Geometry: final body of the model. Coordinates: model frame, mm. Face numbers are marked on the shaded views. A direction names the side the tool comes from. Give positions to 0.01 mm unless a question says otherwise; leave off trailing zeros. Loops run counter-clockwise (first coordinate to the right, second up) from the corner with the lowest first, then second, coordinate; pieces in that order, holes last. Notation, with made-up numbers: (20.5, 40.25) - (69.5, 40.25) arc R16 ccw to (69.5, 63.25) - close; hole circle Ø9 at (55, 82.25). An arc over 180 degrees is marked (long way). Answer in a Markdown table with one row per item.
Solid Edge part; units mm, degrees
sketch "Sketch1" plane through (0, 0, 0) normal (0, -1, 0) x (1, 0, 0)
  circle A0 centre (0, 0) radius 21
extrude "Protrusion1" add sketch "Sketch1" along normal blind 20
sketch "Sketch2" plane through (0, 0, 0) normal (0, -1, 0) x (1, 0, 0)
  circle A0 centre (0, 0) radius 8
extrude "ExtrudedCutout_1" cut sketch "Sketch2" along normal blind 161.3
sketch "Sketch3" plane through (0, 0, 0) normal (0, -1, 0) x (1, 0, 0)
  circle A0 centre (0, 0) radius 16
  circle A1 centre (0, 0) radius 8
extrude "ExtrudedCutout_2" cut sketch "Sketch3" along normal blind 10
sketch "Sketch4" plane through (0, -10, -21) normal (0, 0, -1) x (0, 1, 0)
  circle A0 centre (5, 0) radius 2.5
extrude "Cutout1" cut sketch "Sketch4" against normal up to vertex (21 mm away)
pattern_circular "Pattern1" count 2 over 84.153 about axis through (-0.000024, 0, 0) along (0, 1, 0) of "Cutout1"
sketch "Sketch5" plane through (0, -20, 0) normal (0, -1, 0) x (0, 0, 1)
  circle A0 centre (0, 0) radius 8.35
extrude "Cutout2" cut sketch "Sketch5" against normal blind 63.3
sketch "Sketch6" plane through (-14.849242, -10, -14.849242) normal (-0.7071068, 0, -0.7071068) x (0, 1, 0)
  circle A0 centre (-5, 0) radius 2.25
extrude "ExtrudedCutout_9" cut sketch "Sketch6" against normal blind 20.6
sketch "Sketch7" plane through (-14.849242, -10, -14.849242) normal (-0.7071068, 0, -0.7071068) x (0, 1, 0)
  circle A0 centre (-5, 0) radius 2.25
  circle A1 centre (-5, 0) radius 4.5
extrude "ExtrudedCutout_10" cut sketch "Sketch7" against normal blind 4
chamfer "Chamfer_4" distance 6.98968 angle 45 1 edges at (-21, -20, 0)
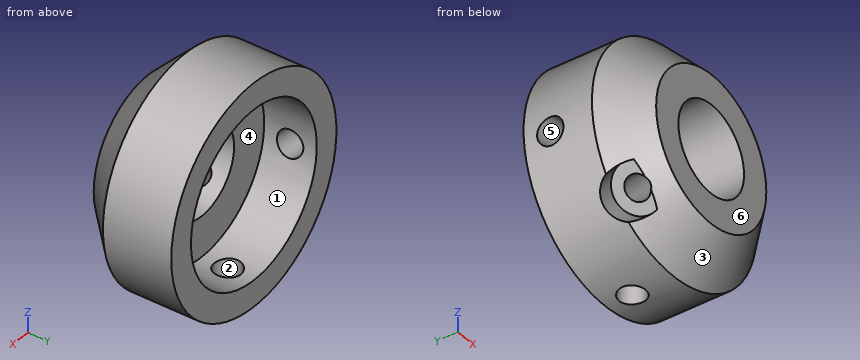
Q1. Cut plane A-A (x = 0). Output: boundary loops of the cut face in (y, z), and give its area (3 significant figures).
Check values:
| item | result |
|---|---|
| outline | (-20, -14.01) - (-13.01, -21) - (-7.5, -21) - (-7.5, -16) - (-10, -16) - (-10, -8.35) - (-20, -8.35) - close; (-20, 8.35) - (-10, 8.35) - (-10, 16) - (0, 16) - (0, 21) - (-13.01, 21) - (-20, 14.01) - close; (-2.5, -21) - (0, -21) - (0, -16) - (-2.5, -16) - close |
| area | 279 mm² |
Q2. Cut plane B-B (y = -5). Output: boundary loops of the cut face in (x, z), and give its area (3 significant figures).
Check values:
| item | result |
|---|---|
| outline | (-21, 0.36) - (-15.98, 0.88) arc R16 cw (long way) to (2.5, -15.8) - (2.5, -20.85) arc R21 ccw (long way) to start; (-20.49, -4.61) arc R21 ccw to (-2.5, -20.85) - (-2.5, -15.8) arc R16 cw to (-15.47, -4.1) - close |
| area | 531 mm² |
Q3. Cut plane D-D (z = 0). Give the number of separate pieces and of enclosed holes in the cut face, and give its area (3 significant figures).
Check values:
| item | result |
|---|---|
| separate pieces | 3 |
| enclosed holes | 0 |
| area | 288 mm² |
Q4. First-contact query: pin 1 (1.5 mm diameter, centred on x = 10.5, y = -12.5, fed in from +Z); pin 2 (16 mm diameter, centred on x = 7.5, z = -1, fed in from +Y); pin 3 (5 mm diameter, centred on y = -4.5, z = 5.5, fed in from -X). Flat tips, straight axial feed; report the tip coordinate or a pass-through.
Check values:
| item | result |
|---|---|
| pin 1 | z = 18.6 |
| pin 2 | y = -10 |
| pin 3 | x = -20.78 |
Q5. Reachability of the marked faces 1, 2 and 3 from +Z, -Z, +X, -X, +Y, -Y: full face, straight path, thin tool, end or side. Return the list, or none.
Check values:
| item | result |
|---|---|
| face 1 | +Y |
| face 2 | -Z |
| face 3 | -Y |
Q6. Draft query along Y for the marked faces 4, 5 and 6. Return one class per face: pulls with the +Y half, pulls with the -Y half, needs draft (parallel to the pull), parting line crosses it, or undercut.
Check values:
| item | result |
|---|---|
| face 4 | pulls with the +Y half |
| face 5 | undercut |
| face 6 | pulls with the -Y half |
Q7. Cut plane C-C (y = -18.5). Output: boundary loops of the cut face in (x, z).
Check values:
| item | result |
|---|---|
| outline | circle Ø31.02 at (0, 0); hole circle Ø16.7 at (0, 0) |
Q8. Material intervals for line 1 along Z through (x, y) = (0, -13); line 2 along Z through (x, y) = (0, -3.25); line 3 along Z through (x, y) = (-12.5, -2.5), sorted ascending.
Check values:
| item | result |
|---|---|
| line 1 | -21 to -8.35, 8.35 to 21 |
| line 2 | 16 to 21 |
| line 3 | -16.87 to -9.99, 9.99 to 16.87 |
